from build123d import *

# Parameters (mm, degrees)
SKETCH_1_W               = 104
SKETCH_1_H               = 40
SKETCH_1_R               = 5
SKETCH_1_R_2             = 1.5
EXTRUDE_1_DEPTH          = 3
SKETCH_2_W               = 5
SKETCH_2_H               = 40
EXTRUDE_2_DEPTH          = 20
CUT_EXTRUDE_1_DEPTH      = 111.431414635
CUT_EXTRUDE_1_DEPTH_BACK = 111.431414635
SKETCH_3_R               = 1.5
SKETCH_3_R_2             = 5
FILLET_1_R               = 10
SKETCH_4_W               = 200
SKETCH_4_H               = 40
EXTRUDE_3_DEPTH          = 100
CUT_EXTRUDE_2_DEPTH      = 100
CUT_EXTRUDE_3_DEPTH      = 185.266376038
CUT_EXTRUDE_3_DEPTH_BACK = 185.266376038
FILLET_2_R               = 5
CUT_EXTRUDE_4_DEPTH      = 226.499661516
CUT_EXTRUDE_4_DEPTH_BACK = 226.499661516
CUT_EXTRUDE_5_DEPTH      = 225.605419664
CUT_EXTRUDE_5_DEPTH_BACK = 225.605419664
SKETCH_8_W               = 135.335857316
SKETCH_8_H               = 8.120151439
SKETCH_9_W               = 20
SKETCH_9_H               = 22
EXTRUDE_4_DEPTH          = 200
CUT_EXTRUDE_6_DEPTH      = 168.657388896
CUT_EXTRUDE_6_DEPTH_BACK = 168.657388896
SKETCH_10_W              = 194
SKETCH_10_H              = 20


with BuildPart() as part:
    # 草图1 → 凸台-拉伸1 (new body)
    with BuildSketch(Plane.XY):
        with Locations((15, 9.156428763)):
            Rectangle(SKETCH_1_W, SKETCH_1_H)
        with Locations((15, 9.156428763)):
            Circle(SKETCH_1_R, mode=Mode.SUBTRACT)
        with Locations((15, 16.656428763)):
            Circle(SKETCH_1_R_2, mode=Mode.SUBTRACT)
        with Locations((22.5, 9.156428763)):
            Circle(SKETCH_1_R_2, mode=Mode.SUBTRACT)
        with Locations((15, 1.656428763)):
            Circle(SKETCH_1_R_2, mode=Mode.SUBTRACT)
        with Locations((7.5, 9.156428763)):
            Circle(SKETCH_1_R_2, mode=Mode.SUBTRACT)
    extrude(amount=EXTRUDE_1_DEPTH)

    # 草图2 → 凸台-拉伸2 (add)
    with BuildSketch(Plane.XY.offset(3)):
        with Locations((-34.5, 9.156428763)):
            Rectangle(SKETCH_2_W, SKETCH_2_H)
        with Locations((64.5, 9.156428763)):
            Rectangle(SKETCH_2_W, SKETCH_2_H)
    extrude(amount=EXTRUDE_2_DEPTH)

    # 草图3 → 切除-拉伸1 (cut, two sides: drawn at the far end of the back side and taken through both)
    with BuildSketch(Plane(origin=(67, 0, 0), x_dir=(0, 0, -1), z_dir=(1, 0, 0)).offset(-CUT_EXTRUDE_1_DEPTH_BACK)):
        with Locations(Location((-13.5, 16.569068444, 0), (0, 0, 90))):
            Circle(SKETCH_3_R)
        with Locations(Location((-13.5, 1.569068444, 0), (0, 0, 90))):
            Circle(SKETCH_3_R)
        with Locations(Location((-13.5, 9.069068444, 0), (0, 0, 90))):
            Circle(SKETCH_3_R_2)
        with Locations(Location((-6, 9.069068444, 0), (0, 0, 90))):
            Circle(SKETCH_3_R)
        with Locations(Location((-21, 9.069068444, 0), (0, 0, 90))):
            Circle(SKETCH_3_R)
    extrude(amount=CUT_EXTRUDE_1_DEPTH + CUT_EXTRUDE_1_DEPTH_BACK, mode=Mode.SUBTRACT)

    # 圆角1
    fillet_1_edges = [part.edges().sort_by_distance(p)[0] for p in [
        (-34.5, 29.156428763, 23),
        (-34.5, -10.843571237, 23),
        (64.5, 29.156428763, 23),
        (64.5, -10.843571237, 23),
    ]]
    fillet(fillet_1_edges, radius=FILLET_1_R)

    # 草图4 → 凸台-拉伸3 (add)
    with BuildSketch(Plane(origin=(0, 0, 0), x_dir=(-1, 0, 0), z_dir=(0, 0, -1))):
        with Locations((-15, 9.156428763)):
            Rectangle(SKETCH_4_W, SKETCH_4_H)
    extrude(amount=EXTRUDE_3_DEPTH)

    # 草图5 → 切除-拉伸2 (cut)
    with BuildSketch(Plane(origin=(0, 29.156428763, 0), x_dir=(1, 0, 0), z_dir=(0, 1, 0))):
        Polygon((112, 97), (-82, 97), (-82, 3), (-32, 3), (-32, -3), (62, -3), (62, 3), (112, 3), align=None)
    extrude(amount=-CUT_EXTRUDE_2_DEPTH, mode=Mode.SUBTRACT)

    # 草图6 → 切除-拉伸3 (cut, two sides: drawn at the far end of the back side and taken through both)
    with BuildSketch(Plane.ZY.offset(37).offset(-CUT_EXTRUDE_3_DEPTH_BACK)):
        Polygon((0, 21.156428763), (22.797958971, 21.156428763), (26.883028225, 31.204196531), (0, 34.707184858), align=None)
        Polygon((0, -2.843571237), (22.797958971, -2.843571237), (28.320151641, -11.460404888), (0, -17.388538979), align=None)
    extrude(amount=CUT_EXTRUDE_3_DEPTH + CUT_EXTRUDE_3_DEPTH_BACK, mode=Mode.SUBTRACT)

    # 圆角2
    fillet_2_edges = [part.edges().sort_by_distance(p)[0] for p in [
        (-34.5, -2.843571237, 22.797958971),
        (-34.5, 21.156428763, 22.797958971),
        (64.5, -2.843571237, 22.797958971),
        (64.5, 21.156428763, 22.797958971),
    ]]
    fillet(fillet_2_edges, radius=FILLET_2_R)

    # 草图7 → 切除-拉伸4 (cut, two sides: drawn at the far end of the back side and taken through both)
    with BuildSketch(Plane.ZY.offset(85).offset(-CUT_EXTRUDE_4_DEPTH_BACK)):
        Polygon((0, 21.156428763), (-100, 21.156428763), (-112.355284076, 36.746993881), (4.033553215, 41.186010001), align=None)
        Polygon((-100, -2.843571237), (0, -2.843571237), (4.033553215, -17.712155102), (-111.164328532, -19.119648018), align=None)
    extrude(amount=CUT_EXTRUDE_4_DEPTH + CUT_EXTRUDE_4_DEPTH_BACK, mode=Mode.SUBTRACT)

    # 草图8 → 切除-拉伸5 (cut, two sides: drawn at the far end of the back side and taken through both)
    with BuildSketch(Plane.ZY.offset(85).offset(-CUT_EXTRUDE_5_DEPTH_BACK)):
        with Locations((-37.649890838, 23.216504482)):
            Rectangle(SKETCH_8_W, SKETCH_8_H)
    extrude(amount=CUT_EXTRUDE_5_DEPTH + CUT_EXTRUDE_5_DEPTH_BACK, mode=Mode.SUBTRACT)

    # 草图9 → 凸台-拉伸4 (add)
    with BuildSketch(Plane.ZY.offset(85)):
        with Locations((-110, 8.156428763)):
            Rectangle(SKETCH_9_W, SKETCH_9_H)
    extrude(amount=-EXTRUDE_4_DEPTH)

    # 草图10 → 切除-拉伸6 (cut, two sides: drawn at the far end of the back side and taken through both)
    with BuildSketch(Plane(origin=(0, 19.156428763, 0), x_dir=(1, 0, 0), z_dir=(0, 1, 0)).offset(-CUT_EXTRUDE_6_DEPTH_BACK)):
        with Locations((15, 107)):
            Rectangle(SKETCH_10_W, SKETCH_10_H)
    extrude(amount=CUT_EXTRUDE_6_DEPTH + CUT_EXTRUDE_6_DEPTH_BACK, mode=Mode.SUBTRACT)


solid = part.part
Input: part model. Units: mm. Frame: model coordinates. A direction names the side the tool comes from. Round coordinates to 2 decimals unless told otherwise and drop trailing zeros. Loops run counter-clockwise (first coordinate to the right, second up) from the corner with the lowest first, then second, coordinate; pieces in that order, holes last. Notation, with made-up numbers: (-11.5, -23) -> (3.5, -23) arc R28 cw to (3.5, 3) -> close; hole circle Ø8 at (-9.75, 82.25). An arc over 180 degrees is marked (long way). Answer as a JSON object with one key per item and string values. Group by question number.
1) Draft query along Y for faces 6 (the flat face through (-85, 8, -61)), 7 (the cylindrical face through (-34.535, 11.376, 9.064)), 8 (the flat face through (15, -2.844, -118)). Return one class per face: +Y half, -Y half, draft (parallel to the pull), parting line (faces both ways), or undercut.
2) Pin query (flat end, axial travel): pin 1 (6.5 mm diameter, centred on x = -67, y = 9.5, fed in from +Z); pin 2 (3.5 mm diameter, centred on y = 1.57, z = 13.5, fed in from +X); pin 3 (8 mm diameter, centred on y = 9.07, z = 13.5, fed in from -X); pin 4 (12 mm diameter, centred on x = -25, y = 0, fed in from +Z). Return the tip coordinate at first contact, or that it passes through.
3) Section query B-B on x = 64. State how many separate pieces and enclosed holes the cut face has, plus the area to 3 significant figures.
4) Section query C-C on x = 23. Output: boundary loops of the cut face in (y, z), plus the area to 3 significant figures.
5) Ray query, L1, parallel to Y at x = -34.6, z = 13.5; L2, parallel to Z at x = 82, y = 16.75; L3, parallel to X at y = 2, z = -12. Return the intervals inside material, ascending.
6) Reachability of faces 1 (the flat face through (-32, 6, 7)), 2 (the flat face through (67, 6, 9)), 3 (the flat face through (-61, 8, 0)), 4 (the flat face through (14, 8, -117)), 5 (the flat face through (115, 8, -61)) from +Z, -Z, +X, -X, +Y, -Y: full face, straight path, thin tool, end or side. Return the list, or none.
7) Section query A-A on z = -18.5. Output: boundary loops of the cut face in (x, y).
Reply:
{
 "1": {"face 6": "draft", "face 7": "undercut", "face 8": "-Y half"},
 "2": {"pin 1": "stops at z = 0", "pin 2": "stops at x = 67", "pin 3": "passes through", "pin 4": "stops at z = -117"},
 "3": {"separate pieces": "2", "enclosed holes": "5", "area": "525 mm2"},
 "4": {"outline": "(-2.84, -120) -> (19.16, -120) -> (19.16, -117) -> (-2.84, -117) -> close", "area": "66.0 mm2"},
 "5": {"L1": "y = -2.84 to 0.07, 3.07 to 4.07, 14.07 to 15.07, 18.07 to 19.16", "L2": "z = -120 to -117, -3 to 0", "L3": "x = -85 to -82, 112 to 115"},
 "6": {"face 1": "+Z, +Y, -Y", "face 2": "+Z, +X, +Y, -Y", "face 3": "+Z, -X, +Y, -Y", "face 4": "+Y, -Y", "face 5": "+Z, -Z, +X, +Y, -Y"},
 "7": {"outline": "(-85, -2.84) -> (-82, -2.84) -> (-82, 19.16) -> (-85, 19.16) -> close; (112, -2.84) -> (115, -2.84) -> (115, 19.16) -> (112, 19.16) -> close"}
}
